from build123d import *

# Parameters (mm, degrees)
BOSS_EXTRUDE1_DEPTH = 4
SKETCH2_OUTSIDE_W   = 20.262
SKETCH2_OUTSIDE_H   = 19.19
SKETCH2_OUTSIDE_R   = 3.464101615
CUT_EXTRUDE1_DEPTH  = 4
CUT_EXTRUDE1_DRAFT  = -45
SKETCH3_R           = 2.25
BOSS_EXTRUDE2_DEPTH = 25


with BuildPart() as part:
    # Sketch1 → Boss-Extrude1 (new body)
    with BuildSketch(Plane.XY):
        Polygon((-2, 3.464101615), (-4, 0), (-2, -3.464101615), (2, -3.464101615), (4, 0), (2, 3.464101615), align=None)
    extrude(amount=BOSS_EXTRUDE1_DEPTH)


with BuildPart() as cut_extrude1_tool:
    # Sketch2 outside → Cut-Extrude1 (with draft: the straight prism first)
    with BuildSketch(Plane.XY.offset(4)):
        Rectangle(SKETCH2_OUTSIDE_W, SKETCH2_OUTSIDE_H)
        Circle(SKETCH2_OUTSIDE_R, mode=Mode.SUBTRACT)
    extrude(amount=-CUT_EXTRUDE1_DEPTH)
    # Cut-Extrude1: the draft: its side faces are tilted about the plane it starts from
    cut_extrude1_sides = [cut_extrude1_tool.faces().sort_by_distance(p)[0] for p in [
        (0, -9.595, 2),
        (10.131, 0, 2),
        (0, 9.595, 2),
        (-10.131, 0, 2),
        (-3.464101615, 0, 2),
    ]]
    draft(cut_extrude1_sides, Plane.XY.offset(4), CUT_EXTRUDE1_DRAFT)


with BuildPart() as part_1:
    add(part.part)

    # Cut-Extrude1: cut by cut_extrude1_tool
    add(cut_extrude1_tool.part, mode=Mode.SUBTRACT)

    # Sketch3 → Boss-Extrude2 (add)
    with BuildSketch(Plane(origin=(0, 0, 0), x_dir=(-1, 0, 0), z_dir=(0, 0, -1))):
        Circle(SKETCH3_R)
    extrude(amount=BOSS_EXTRUDE2_DEPTH)


solid = part_1.part
The model under review builds one solid part; all positions refer to its coordinate system, in mm. A direction names the side the tool comes from. Round coordinates to 2 decimals unless told otherwise and drop trailing zeros. Loops run counter-clockwise (first coordinate to the right, second up) from the corner with the lowest first, then second, coordinate; pieces in that order, holes last. Notation, with made-up numbers: (38.5, -14.75) -> (52.5, -14.75) arc R17 ccw to (52.5, -1.75) -> close; hole circle Ø6 at (9.5, -30.5). An arc over 180 degrees is marked (long way). Write item = value, one per line. Start each with the question number.
Item 1: Insertion check: pin 1 (3 mm diameter, centred on y = 0, z = -4.5, fed in from +X); pin 2 (3 mm diameter, centred on x = 0.5, z = -19.5, fed in from +Y); pin 3 (3 mm diameter, centred on x = 2.5, z = -10, fed in from +Y). Each pin has a flat end and moves straight along its axis. Give the tip position at first contact, or say it passes through.
Item 2: Take a section at A-A on z = -15. Give the boundary of the cut face in (x, y), plus the area to 3 significant figures.
Item 3: For faces 1 (the flat face through (2, 2, 0)), 2 (the conical face through (3.592, -0.009, 3.872)), list the 3-axis set-ups (+Z, -Z, +X, -X, +Y, -Y) from which the entire face can be reached by the end or side of a thin tool; tool diameter is ignored.
Item 4: To check wall thickness, follow L1, parallel to Z at x = 1.75, y = -2.5; L2, parallel to Y at x = 3, z = 0.5; L3, parallel to Y at x = 0, z = -1. State the ranges of each line that lie inside material, in increasing order.
Result:
q1.pin_1 = 2.25
q1.pin_2 = 2.25
q1.pin_3 = 2.02
q2.outline = circle Ø4.5 at (0, 0)
q2.area = 15.9 mm²
q3.face_1 = -Z
q3.face_2 = +Z, +X
q4.L1 = 0 to 4
q4.L2 = -1.73 to 1.73
q4.L3 = -2.25 to 2.25
